Could you check a few things on this model? Use its own coordinates, in mm. Round coordinates to 2 decimals unless told otherwise and drop trailing zeros. Order: outer loops, then holes, each group sorted by start corner. A loop starts at its lowest first (then second) coordinate and runs counter-clockwise, first axis right, second up. Notation, with made-up numbers: (-30, 61) - (-23, 61) arc R16 cw to (-23, 72) - close; hole circle Ø1 at (77.25, 82.5). An arc over 180 degrees is marked (long way). Return JSON: item names as keys, results as strings. Group by question number.
from build123d import *

# Parameters (mm, degrees)
BOSS_EXTRUDE1_START = -0.5
BOSS_EXTRUDE1_DEPTH = 0.5
CUT_EXTRUDE1_DEPTH  = 0.5
CIRPATTERN2_COUNT   = 4


with BuildPart() as part:
    # Sketch1 → Revolve1 (revolve)
    with BuildSketch(Plane.XY):
        with BuildLine():
            Line((-32.130708731, -1), (-34, 0))
            ThreePointArc((-34, 0), (-35, -1), (-34, -2))
            Line((-34, -2), (-32, -14))
            Line((-32, -14), (-20, -77))
            Line((-20, -77), (-12.6, -77))
            Line((-12.6, -77), (-12.6, -75.5))
            Line((-12.6, -75.5), (0, -75.5))
            Line((0, -75.5), (0, -74))
            Line((0, -74), (-18.535470636, -74))
            Line((-18.535470636, -74), (-29.964042064, -14))
            Line((-29.964042064, -14), (-32.130708731, -1))
        make_face()
    revolve(axis=Axis((0, 0, 0), (0, -1, 0)))

    # Sketch3 → Boss-Extrude1 (add)
    with BuildSketch(Plane.XZ.offset(77).offset(BOSS_EXTRUDE1_START)):
        with BuildLine():
            Line((-0.25, 12.597519597), (-0.25, 11.997519597))
            Line((-0.25, 11.997519597), (0.25, 11.997519597))
            Line((0.25, 11.997519597), (0.25, 12.597519597))
            ThreePointArc((0.25, 12.597519597), (0, 12.6), (-0.25, 12.597519597))
        make_face()
    boss_extrude1 = extrude(amount=BOSS_EXTRUDE1_DEPTH)

    # Sketch8 → Cut-Extrude1 (cut)
    with BuildSketch(Plane.ZY.offset(0.25)):
        Polygon((11.997519597, -76.75), (12.597519597, -77), (11.997519597, -77), align=None)
    cut_extrude1 = extrude(amount=-CUT_EXTRUDE1_DEPTH, mode=Mode.SUBTRACT)

    # CirPattern2: Boss-Extrude1, Cut-Extrude1 ×4 about axis
    cirpattern2_axis = Axis((0, 0, 0), (0, 1, 0))
    add([boss_extrude1.rotate(cirpattern2_axis, i * 360 / CIRPATTERN2_COUNT) for i in range(1, CIRPATTERN2_COUNT)])
    add([cut_extrude1.rotate(cirpattern2_axis, i * 360 / CIRPATTERN2_COUNT) for i in range(1, CIRPATTERN2_COUNT)], mode=Mode.SUBTRACT)


solid = part.part
1) I want a section at B-B, the plane y = -57. List the corners of the cut face in (x, z) for me.
2) Will these pins go through, and if not, where does the flat tip stop? pin 1 (12 mm diameter, centred on x = -25.5, y = -65.5, fed in from +Z); pin 2 (8 mm diameter, centred on x = -2, y = -49.5, fed in from -Z); pin 3 (0.6 mm diameter, centred on x = -12.5, y = -77, fed in from +Z).
3) I want a section at A-A, the plane y = -23. List the corners of the cut face in (x, z) for me.
4) We'd pull the mould along X, two halves only. Please class faces 1 (the flat face through (0, -74, 0)), 2 (the conical face through (5.33, -52.94, 24)), 3 (the flat face through (13, -77, 0)): +X half, -X half, draft (parallel to the pull), parting line (faces both ways), or undercut.
5) If I drill on line 1 along Z through (x, y) = (0, -14); line 2 along Z through (x, y) = (0, -75.9); line 3 along X through (y, z) = (-62.5, 10), over which ranges is the centre line in solid material (lowest first)? Write a range as from..to.
Outcome:
{
 "1": {"outline": "circle Ø47.62 at (0, 0); hole circle Ø43.55 at (0, 0)"},
 "2": {"pin 1": "z = 10.85", "pin 2": "z = -25.96", "pin 3": "z = 15.86"},
 "3": {"outline": "circle Ø60.57 at (0, 0); hole circle Ø56.5 at (0, 0)"},
 "4": {"face 1": "undercut", "face 2": "parting line", "face 3": "draft"},
 "5": {"line 1": "-32..-29.96, 29.96..32", "line 2": "-20.21..-12.6, 12.6..20.21", "line 3": "-20.45..-18.15, 18.15..20.45"}
}
